Source: CAD feature listing. Evaluate the final solid. Frame: model axes, mm. A direction names the side the tool comes from. Round coordinates to 2 decimals unless told otherwise and drop trailing zeros. Write each loop counter-clockwise with the first axis right and the second up, starting at its lowest first coordinate (ties: lowest second). Pieces come first, ordered by that corner, then holes. Notation, with made-up numbers: M 70,35 L 101,35 A12 ccw 101,45 Z; hole C 32,-5 d7. An arc over 180 degrees is marked long. Answer in a Markdown table with one row per item.
from build123d import *

# Parameters (mm, degrees)
SKETCH2_W           = 100
SKETCH2_H           = 50
BOSS_EXTRUDE1_DEPTH = 3
BOSS_EXTRUDE2_DEPTH = 60


with BuildPart() as part:
    # Sketch2 → Boss-Extrude1 (new body)
    with BuildSketch(Plane(origin=(0, 0, 0), x_dir=(1, 0, 0), z_dir=(0, 1, 0))):
        Rectangle(SKETCH2_W, SKETCH2_H)
    extrude(amount=-BOSS_EXTRUDE1_DEPTH)

    # Sketch3 → Boss-Extrude2 (add)
    with BuildSketch(Plane(origin=(50, 0, 0), x_dir=(0, 0, -1), z_dir=(1, 0, 0))):
        Polygon((25, 0), (67.426406871, 42.426406871), (67.426406871, 39.426406871), (25, -3), align=None)
    extrude(amount=-BOSS_EXTRUDE2_DEPTH)


solid = part.part
Q1. Section B-B (z = 5.5). Return loops of the section in (x, y).
Solutions:
| item | result |
|---|---|
| outline | M -50,-3 L 50,-3 L 50,0 L -50,0 Z |
Q2. Material intervals for probe 1 along Y at (x, z) = (-29.5, -12.5); probe 2 along Z at (x, y) = (-1, 21); probe 3 along Y at (x, z) = (24, -39), sorted ascending.
Solutions:
| item | result |
|---|---|
| probe 1 | y = -3 to 0 |
| probe 2 | z = -49 to -46 |
| probe 3 | y = 11 to 14 |
Q3. Contact query for flat-ended pins moving along their axis: pin 1 Ø3 at (x, z) = (38, 7.5) entering from +Y; pin 2 Ø3.5 at (x, y) = (-33, -2) entering from -Z; pin 3 Ø1.5 at (x, y) = (2.5, 11) entering from +Z. Output: stop coordinate, or through.
Solutions:
| item | result |
|---|---|
| pin 1 | stops at y = 0 |
| pin 2 | stops at z = -25 |
| pin 3 | stops at z = -35.25 |
Q4. Section A-A (x = 8). Return loops of the section in (y, z), and give its area (3 significant figures).
Solutions:
| item | result |
|---|---|
| outline | M -3,-25 L 39.43,-67.43 L 42.43,-67.43 L 0,-25 L 0,25 L -3,25 Z |
| area | 277 mm2 |
Q5. Section C-C (y = 34.5). Return loops of the section in (x, z), and give its area (3 significant figures).
Solutions:
| item | result |
|---|---|
| outline | M -10,-62.5 L 50,-62.5 L 50,-59.5 L -10,-59.5 Z |
| area | 180 mm2 |
Q6. Access query for faces 1 (the flat face through (-1, -1, 25)), 2 (the flat face through (-1, 0, 0)), 3 (the flat face through (-30, -1, -25)). Directions: +Z, -Z, +X, -X, +Y, -Y. A direction counts if a zero-diameter tool reaches every point of the face in a straight line with its end or side. Return the directions, or none.
Solutions:
| item | result |
|---|---|
| face 1 | +Z, +X, -X, +Y, -Y |
| face 2 | +Z, +X, -X, +Y |
| face 3 | -Z, -X, +Y, -Y |
